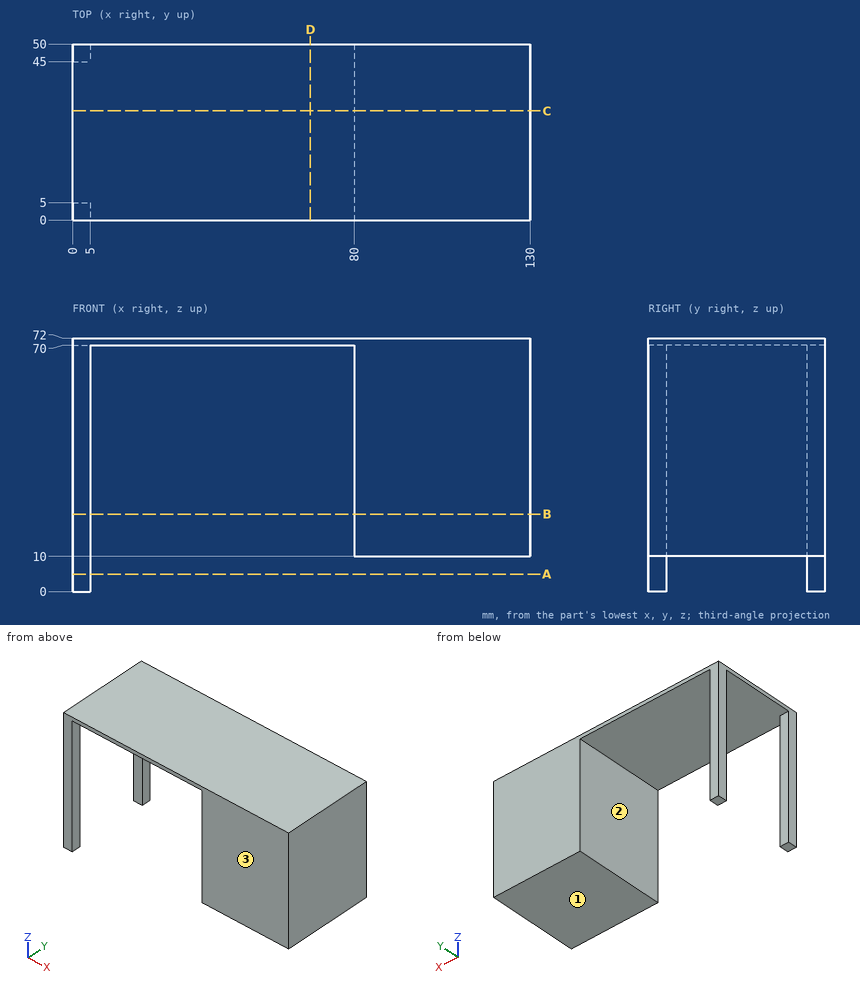
Input: dimensioned drawing with shaded views. Units: mm. Origin: part minimum x, y, z. A direction names the side the tool comes from. Round coordinates to 2 decimals unless told otherwise and drop trailing zeros. Loops run counter-clockwise (first coordinate to the right, second up) from the corner with the lowest first, then second, coordinate; pieces in that order, holes last. Notation, with made-up numbers: (83.5, 22) -> (90.5, 22) arc R27 ccw to (90.5, 51) -> close; hole circle Ø5 at (-1.75, 38). An arc over 180 degrees is marked (long way). Use one line per item in the form item = value. Start each with the question number.
1) First-contact query: P1, Ø3, axis at y = 31.5, z = 48.5, coming from the -X side; P2, Ø25, axis at x = 96, y = 17.5, coming from the -Z side. Flat tips, straight axial feed; report the tip coordinate or a pass-through.
2) Section B-B on z = 22. Output: boundary loops of the cut face in (x, y), then the cut area to 3 significant figures.
3) Section C-C on y = 31. Output: boundary loops of the cut face in (x, z), then the cut area to 3 significant figures.
4) Section A-A on z = 5. Output: boundary loops of the cut face in (x, y), then the cut area to 3 significant figures.
5) Access query for the marked faces 1, 2 and 3. Directions: +Z, -Z, +X, -X, +Y, -Y. A direction counts if a zero-diameter tool reaches every point of the face in a straight line with its end or side. Return the directions, or none.
6) Line query: L1, parallel to X at y = 3.5, z = 39; L2, parallel to Z at x = 113, y = 29; L3, parallel to Z at x = 77, y = 47. Output: solid intervals per line, ascending.
7) Section D-D on x = 67.5. Output: boundary loops of the cut face in (y, z).
Response:
q1.P1 = 80
q1.P2 = 10
q2.outline = (0, 0) -> (5, 0) -> (5, 5) -> (0, 5) -> close; (0, 45) -> (5, 45) -> (5, 50) -> (0, 50) -> close; (80, 0) -> (130, 0) -> (130, 50) -> (80, 50) -> close
q2.area = 2,550 mm^2
q3.outline = (0, 70) -> (80, 70) -> (80, 10) -> (130, 10) -> (130, 72) -> (0, 72) -> close
q3.area = 3,260 mm^2
q4.outline = (0, 0) -> (5, 0) -> (5, 5) -> (0, 5) -> close; (0, 45) -> (5, 45) -> (5, 50) -> (0, 50) -> close
q4.area = 50.0 mm^2
q5.face_1 = -Z, +X, +Y, -Y
q5.face_2 = -Z, +Y, -Y
q5.face_3 = +Z, -Z, +X, -X, -Y
q6.L1 = 0 to 5, 80 to 130
q6.L2 = 10 to 72
q6.L3 = 70 to 72
q7.outline = (0, 70) -> (50, 70) -> (50, 72) -> (0, 72) -> close
